The model under review builds one solid part; all positions refer to its coordinate system, in mm. A direction names the side the tool comes from. Give positions to 0.01 mm unless a question says otherwise; leave off trailing zeros. Order: outer loops, then holes, each group sorted by start corner. A loop starts at its lowest first (then second) coordinate and runs counter-clockwise, first axis right, second up. Notation, with made-up numbers: (-15.75, 40) - (15.25, 40) arc R20 ccw to (15.25, 71) - close; hole circle Ø4 at (84.5, 82.5). An arc over 180 degrees is marked (long way). Use CSV: the item, a comma, the result in double quotes.
```python
from build123d import *

# Parameters (mm, degrees)
PAD012_DEPTH    = 1.5
SKETCH014_R     = 1.7
POCKET004_DEPTH = 1.501
SKETCH015_W     = 104
SKETCH015_H     = 75
PAD011_DEPTH    = 1.5
SKETCH016_W     = 89
SKETCH016_H     = 68
POCKET005_DEPTH = 0.01
SKETCH019_W     = 20
SKETCH019_H     = 18
PAD010_DEPTH    = 6
SKETCH018_R     = 2.75
SKETCH018_R_2   = 1.7
PAD009_DEPTH    = 15


with BuildPart() as part:
    # Sketch017 → Pad012 (new body)
    with BuildSketch(Plane.XY):
        with BuildLine():
            Line((3.5, 75), (114.5, 75))
            ThreePointArc((118, 71.5), (116.9748737342, 73.9748737342), (114.5, 75))
            Line((118, 71.5), (118, 3.5))
            ThreePointArc((114.5, 0), (116.9748737342, 1.0251262658), (118, 3.5))
            Line((114.5, 0), (3.5, 0))
            ThreePointArc((0, 3.5), (1.0251262658, 1.0251262658), (3.5, 0))
            Line((0, 3.5), (0, 71.5))
            ThreePointArc((3.5, 75), (1.0251262658, 73.9748737342), (0, 71.5))
        make_face()
    extrude(amount=PAD012_DEPTH)

    # Sketch014 (on Face10 of Pad012) → Pocket004 (cut, through all)
    with BuildSketch(Plane.XY.offset(1.5)):
        with Locations((3.5, 3.5)):
            Circle(SKETCH014_R)
        with Locations((3.5, 71.5)):
            Circle(SKETCH014_R)
        with Locations((114.5, 71.5)):
            Circle(SKETCH014_R)
        with Locations((114.5, 3.5)):
            Circle(SKETCH014_R)
    extrude(amount=-POCKET004_DEPTH, mode=Mode.SUBTRACT)

    # Sketch015 (on Face5 of Pocket004) → Pad011 (join)
    with BuildSketch(Plane.XY.offset(1.5)):
        with Locations((59, 37.5)):
            Rectangle(SKETCH015_W, SKETCH015_H)
    extrude(amount=PAD011_DEPTH)

    # Sketch016 (on Face19 of Pad011) → Pocket005 (cut)
    with BuildSketch(Plane.XY.offset(3)):
        with Locations((62.5, 37.5)):
            Rectangle(SKETCH016_W, SKETCH016_H)
    extrude(amount=-POCKET005_DEPTH, mode=Mode.SUBTRACT)

    # Sketch019 (on Face4 of Pocket005) → Pad010 (join)
    with BuildSketch(Plane(origin=(0, 0, 0), x_dir=(1, 0, 0), z_dir=(0, 0, -1))):
        with Locations((123, -37.5)):
            Rectangle(SKETCH019_W, SKETCH019_H)
    extrude(amount=PAD010_DEPTH)

    # Sketch018 (on Face4 of Pad010) → Pad009 (join)
    with BuildSketch(Plane(origin=(0, 0, 0), x_dir=(1, 0, 0), z_dir=(0, 0, -1))):
        with Locations((3.5, -3.5)):
            Circle(SKETCH018_R)
        with Locations((3.5, -3.5)):
            Circle(SKETCH018_R_2, mode=Mode.SUBTRACT)
        with Locations((114.5, -3.5)):
            Circle(SKETCH018_R)
        with Locations((114.5, -3.5)):
            Circle(SKETCH018_R_2, mode=Mode.SUBTRACT)
        with Locations((114.5, -71.5)):
            Circle(SKETCH018_R)
        with Locations((114.5, -71.5)):
            Circle(SKETCH018_R_2, mode=Mode.SUBTRACT)
        with Locations((3.5, -71.5)):
            Circle(SKETCH018_R)
        with Locations((3.5, -71.5)):
            Circle(SKETCH018_R_2, mode=Mode.SUBTRACT)
    extrude(amount=PAD009_DEPTH)


with BuildPart() as part_1:
    # Body002 placement: moved
    add(part.part.moved(Location((-62.5, -37.5, 19))))


solid = part_1.part
```
Item 1: Take a section at A-A, the plane z = 7.25. Give the boundary of the cut face in (x, y), and give its area (3 significant figures).
Results list:
outline,"circle Ø5.5 at (-59, -34); circle Ø5.5 at (-59, 34); circle Ø5.5 at (52, -34); circle Ø5.5 at (52, 34); hole circle Ø3.4 at (-59, -34); hole circle Ø3.4 at (-59, 34); hole circle Ø3.4 at (52, -34); hole circle Ø3.4 at (52, 34)"
area,"58.7 mm2"
Item 2: Mouldability with a two-part tool opening along Y and no side actions: class faces 1 (the face through (-61.027, -35.859, 11.605)), 2 (the face through (54, -34, 4)), 3 (the face through (-3, -37.5, 20)) as pulls with the +Y half, pulls with the -Y half, needs draft (parallel to the pull), parting line crosses it, or undercut.
Results list:
face 1,"undercut"
face 2,"needs draft"
face 3,"pulls with the -Y half"
Item 3: Wall thickness on L1, parallel to Y at x = -59, z = 10.75; L2, parallel to X at y = 34, z = 15.75; L3, parallel to Y at x = 52, z = 19.6: over which ranges is each line inside the solid? List them lowest first.
Results list:
L1,"y = -36.75 to -35.7, -32.3 to -31.25, 31.25 to 32.3, 35.7 to 36.75"
L2,"x = -61.75 to -60.7, -57.3 to -56.25, 49.25 to 50.3, 53.7 to 54.75"
L3,"y = -37.5 to -35.7, -32.3 to 32.3, 35.7 to 37.5"
Item 4: Take a section at B-B, the plane z = 14.5. State how many separate pieces and enclosed holes the cut face has, and give its area (3 significant figures).
Results list:
separate pieces,"5"
enclosed holes,"4"
area,"419 mm2"
Item 5: Clearance check with flat-ended pins moving along their axes: pin 1 (2 mm diameter, centred on x = -59.5, y = 17, fed in from +Z); pin 2 (7.5 mm diameter, centred on x = 61.5, y = -3, fed in from +Z); pin 3 (3 mm diameter, centred on y = 3.5, z = 16, fed in from -X); pin 4 (5 mm diameter, centred on x = 46.5, z = 6.5, fed in from -Y). State where each tip first meets the part, or that it passes through.
Results list:
pin 1,"stops at z = 20.5"
pin 2,"stops at z = 19"
pin 3,"stops at x = 50.5"
pin 4,"passes through"
Item 6: Tool access review of faces 4 (the face through (-61.027, 32.141, 11.605)), 5 (the face through (-59, 1, 20.5)), 6 (the face through (60, -9, 16)): name each direction out of +Z, -Z, +X, -X, +Y, -Y from which nothing blocks a thin tool from reaching the whole face with its end or side.
Results list:
face 4,"-Z"
face 5,"+Z, -X, +Y, -Y"
face 6,"-Z, +X, -X"
